Read the model definition and answer for the solid it produces. Units are mm, in the model's axes. A direction names the side the tool comes from. Round coordinates to 2 decimals unless told otherwise and drop trailing zeros. Order: outer loops, then holes, each group sorted by start corner. A loop starts at its lowest first (then second) coordinate and runs counter-clockwise, first axis right, second up. Notation, with made-up numbers: (65, 17.25) -> (114, 17.25) arc R18 cw to (114, 46.25) -> close; hole circle Ø9 at (-24, 56.5). An arc over 180 degrees is marked (long way). Answer as a JSON object with one key per item and string values. Group by question number.
Item 1: Section A-A, the plane x = 2.5 is taken. Count the separate pieces of the cut face and the enclosed holes in it, plus the area to 3 significant figures.
Item 2: Consider probe 1 along Y at (x, z) = (28.95, 48.9); probe 2 along Y at (x, z) = (11.5, 49); probe 3 along Z at (x, y) = (6, 27.5). Determine where each line is inside the solid, lowest interval first. Write a range as from..to.
Item 3: For faces 4 (the flat face through (-19.5, 23, 89)), 5 (the flat face through (-5, 27, 51)), 6 (the cylindrical face through (2.54, 24.82, 11.51)), determine the directions among +Z, -Z, +X, -X, +Y, -Y from which every point of the face is accessible in a straight line to the end or side of a thin tool.
Item 4: Section C-C, the plane z = 114 is taken. Write down the section's boundary in (x, y).
Item 5: The mould has two halves that part along Z. Classify faces 1 (the flat face through (20, 15, 46)), 2 (the flat face through (9.3, 32, 77.9)), 3 (the cylindrical face through (2.54, 16.57, 2.15)): pulls with the +Z half, pulls with the -Z half, needs draft (parallel to the pull), parting line crosses it, or undercut.
Item 6: Section D-D, the plane x = -23.95 is taken. Write down the section's boundary in (y, z).
Item 7: Given P1, Ø4, axis at y = 15, z = 19.2, coming from the +X side; P2, Ø2.5, axis at y = 15, z = 2.8, coming from the -X side; P3, Ø5, axis at x = -14.01, z = 68, coming from the -Y side; P4, Ø3.5, axis at x = -14.01, z = 103, coming from the +Y side, each flat-ended and moving along its own axis, determine where each tip first touches the part or whether it passes through.
from build123d import *

# Parameters (mm, degrees)
BOX001_W        = 65
BOX001_H        = 34
BOX001_DEPTH    = 5
BOX_W           = 5
BOX_H           = 34
BOX_DEPTH       = 46
SKETCH_R        = 2.05
POCKET_DEPTH    = 5
SKETCH001_R     = 5
SKETCH001_R_2   = 1.7
POCKET001_DEPTH = 5
BOX002_W        = 44
BOX002_H        = 17
BOX002_DEPTH    = 78
SKETCH003_R     = 4
SKETCH003_R_2   = 1.5
POCKET003_DEPTH = 17.001
SKETCH008_R     = 10
POCKET006_DEPTH = 34.001


with BuildPart() as cubo001:
    # Box001 → Box001 (new body)
    with BuildSketch(Plane(origin=(-30, -2, 46), x_dir=(1, 0, 0), z_dir=(0, 0, 1))):
        with Locations((32.5, 17)):
            Rectangle(BOX001_W, BOX001_H)
    extrude(amount=BOX001_DEPTH)


with BuildPart() as pocket001:
    # Box → Box (new body)
    with BuildSketch(Plane(origin=(0, -2, 0), x_dir=(1, 0, 0), z_dir=(0, 0, 1))):
        with Locations((2.5, 17)):
            Rectangle(BOX_W, BOX_H)
    extrude(amount=BOX_DEPTH)

    # Fusion: union Cubo001
    add(cubo001.part)

    # Sketch → Pocket (cut)
    with BuildSketch(Plane.XY.offset(51)):
        with Locations((-36.05, -7.05)):
            Circle(SKETCH_R)
        with Locations((28.95, 3.05)):
            Circle(SKETCH_R)
        with Locations((-55.15, -7.05)):
            Circle(SKETCH_R)
        with Locations((9.85, 3.05)):
            Circle(SKETCH_R)
        with Locations((-4.85, 3.05)):
            Circle(SKETCH_R)
        with Locations((-23.95, 3.05)):
            Circle(SKETCH_R)
        with Locations((-23.95, 26.95)):
            Circle(SKETCH_R)
        with Locations((-4.85, 26.95)):
            Circle(SKETCH_R)
        with Locations((9.85, 26.95)):
            Circle(SKETCH_R)
        with Locations((28.95, 26.95)):
            Circle(SKETCH_R)
    extrude(amount=-POCKET_DEPTH, mode=Mode.SUBTRACT)

    # Sketch001 → Pocket001 (cut)
    with BuildSketch(Plane.YZ.offset(5)):
        with Locations((15, 11)):
            Circle(SKETCH001_R)
        with Locations((15, 19.2)):
            Circle(SKETCH001_R_2)
        with Locations((23.2, 11)):
            Circle(SKETCH001_R_2)
        with Locations((15, 2.8)):
            Circle(SKETCH001_R_2)
        with Locations((6.8, 11)):
            Circle(SKETCH001_R_2)
    extrude(amount=-POCKET001_DEPTH, mode=Mode.SUBTRACT)


with BuildPart() as pocket006:
    # Box002 → Box002 (new body)
    with BuildSketch(Plane(origin=(-19.5, 15, 51), x_dir=(1, 0, 0), z_dir=(0, 0, 1))):
        with Locations((22, 8.5)):
            Rectangle(BOX002_W, BOX002_H)
    extrude(amount=BOX002_DEPTH)

    # Sketch003 → Pocket003 (cut, through all)
    with BuildSketch(Plane(origin=(-19.5, 15, 51), x_dir=(1, 0, 0), z_dir=(0, -1, 0))):
        with Locations((22, 6)):
            Circle(SKETCH003_R)
        with Locations((22, 63)):
            Circle(SKETCH003_R)
        with Locations((5.485017, 17)):
            Circle(SKETCH003_R_2)
        with Locations((38.514983, 17)):
            Circle(SKETCH003_R_2)
        with Locations((5.485017, 52)):
            Circle(SKETCH003_R_2)
        with Locations((38.514983, 52)):
            Circle(SKETCH003_R_2)
    extrude(amount=-POCKET003_DEPTH, mode=Mode.SUBTRACT)

    # Fusion001003: union Pocket001
    add(pocket001.part)

    # Sketch008 → Pocket006 (cut, through all)
    with BuildSketch(Plane(origin=(0, 32, 0), x_dir=(-1, 0, 0), z_dir=(0, 1, 0))):
        with Locations((-2.500008, 85.500008)):
            Circle(SKETCH008_R)
    extrude(amount=-POCKET006_DEPTH, mode=Mode.SUBTRACT)


solid = pocket006.part
Values found:
{
 "1": {"separate pieces": "4", "enclosed holes": "5", "area": "2,330 mm2"},
 "2": {"probe 1": "-2..1, 5.1..24.9, 29..32", "probe 2": "-2..1.83, 4.27..25.73, 28.17..32", "probe 3": "46..55.06, 58.94..76.13, 94.87..112.06, 115.94..129"},
 "3": {"face 4": "+Z, -X, +Y, -Y", "face 5": "-Z", "face 6": "+X, -X"},
 "4": {"outline": "(-19.5, 15) -> (-1.5, 15) -> (-1.5, 32) -> (-19.5, 32) -> close; (6.5, 15) -> (24.5, 15) -> (24.5, 32) -> (6.5, 32) -> close"},
 "5": {"face 1": "pulls with the -Z half", "face 2": "needs draft", "face 3": "undercut"},
 "6": {"outline": "(-2, 46) -> (1, 46) -> (1, 51) -> (-2, 51) -> close; (5.1, 46) -> (24.9, 46) -> (24.9, 51) -> (5.1, 51) -> close; (29, 46) -> (32, 46) -> (32, 51) -> (29, 51) -> close"},
 "7": {"P1": "x = 5", "P2": "through", "P3": "y = 15", "P4": "y = 32"}
}
